```python
from build123d import *

# Parameters (mm, degrees)
SKETCH_1_R          = 5
EXTRUDE_1_DEPTH     = 10
SKETCH_2_R          = 3
EXTRUDE_2_DEPTH     = 10
SKETCH_3_R          = 2
CUT_EXTRUDE_1_DEPTH = 10


with BuildPart() as part:
    # 草图1 → 凸台-拉伸1 (new body)
    with BuildSketch(Plane(origin=(0, 0, 0), x_dir=(1, 0, 0), z_dir=(0, 1, 0))):
        with Locations(Location((0, 0, 0), (0, 0, 270))):
            Circle(SKETCH_1_R)
    extrude(amount=EXTRUDE_1_DEPTH)

    # 草图2 → 凸台-拉伸2 (add)
    with BuildSketch(Plane(origin=(0, 10, 0), x_dir=(1, 0, 0), z_dir=(0, 1, 0))):
        with Locations(Location((0, 0, 0), (0, 0, 270))):
            Circle(SKETCH_2_R)
    extrude(amount=EXTRUDE_2_DEPTH)

    # 草图3 → 切除-拉伸1 (cut)
    with BuildSketch(Plane(origin=(0, 20, 0), x_dir=(1, 0, 0), z_dir=(0, 1, 0))):
        with Locations(Location((0, 0, 0), (0, 0, 270))):
            Circle(SKETCH_3_R)
    extrude(amount=-CUT_EXTRUDE_1_DEPTH, mode=Mode.SUBTRACT)


solid = part.part
```
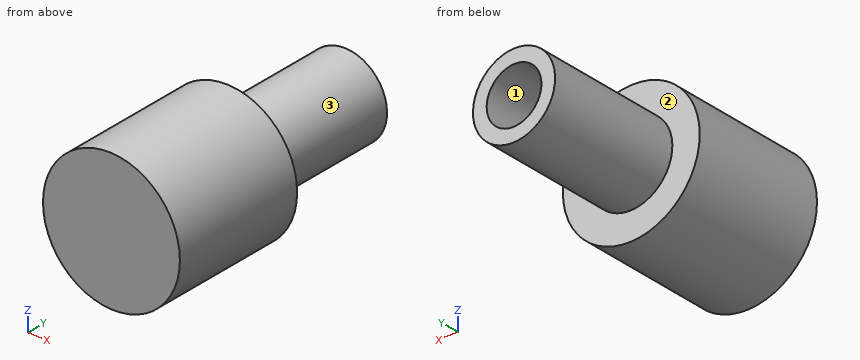
Build history of the part. All positions in model axes, mm. Face numbers are marked on the shaded views. Round coordinates to 2 decimals unless told otherwise and drop trailing zeros. Write each loop counter-clockwise with the first axis right and the second up, starting at its lowest first coordinate (ties: lowest second). Pieces come first, ordered by that corner, then holes.
1) Band-saw the part on A-A, the plane x = 0. List the corners of the cut face in (y, z), and give its area (3 significant figures).
2) Band-saw the part on D-D, the plane y = 2. List the corners of the cut face in (x, z).
3) Mould opens along X. For the marked faces 1, 2 and 3 say: +X half, -X half, draft (parallel to the pull), parting line (faces both ways), or undercut.
4) Band-saw the part on C-C, the plane z = 0. List the corners of the cut face in (x, y), and give its area (3 significant figures).
5) Pin check, flat tips, straight feed: pin 1 (3.5 mm diameter, centred on x = 0, z = 0, fed in from +Y); pin 2 (1 mm diameter, centred on x = 2, y = 5.5, fed in from +Z); pin 3 (6 mm diameter, centred on y = 11.5, z = -3.5, fed in from +X). Stop position of each tip, or through.
6) Drill centre lines: probe 1 along X at (y, z) = (14.5, 0); probe 2 along Y at (x, z) = (1.75, -3.25); probe 3 along X at (y, z) = (16.5, 1.25). Where is each one in solid material? Low to high.
7) Band-saw the part on B-B, the plane y = 11.5. List the corners of the cut face in (x, z), and give its area (3 significant figures).
Ans:
1. outline: (0, -5) - (10, -5) - (10, -3) - (20, -3) - (20, -2) - (10, -2) - (10, 2) - (20, 2) - (20, 3) - (10, 3) - (10, 5) - (0, 5) - close
1. area: 120 mm2
2. outline: circle Ø10 at (0, 0)
3. face 1: undercut
3. face 2: draft
3. face 3: parting line
4. outline: (-5, 0) - (5, 0) - (5, 10) - (3, 10) - (3, 20) - (2, 20) - (2, 10) - (-2, 10) - (-2, 20) - (-3, 20) - (-3, 10) - (-5, 10) - close
4. area: 120 mm2
5. pin 1: stops at y = 10
5. pin 2: stops at z = 4.77
5. pin 3: stops at x = 4.92
6. probe 1: x = -3 to -2, 2 to 3
6. probe 2: y = 0 to 10
6. probe 3: x = -2.73 to -1.56, 1.56 to 2.73
7. outline: circle Ø6 at (0, 0); hole circle Ø4 at (0, 0)
7. area: 15.7 mm2
